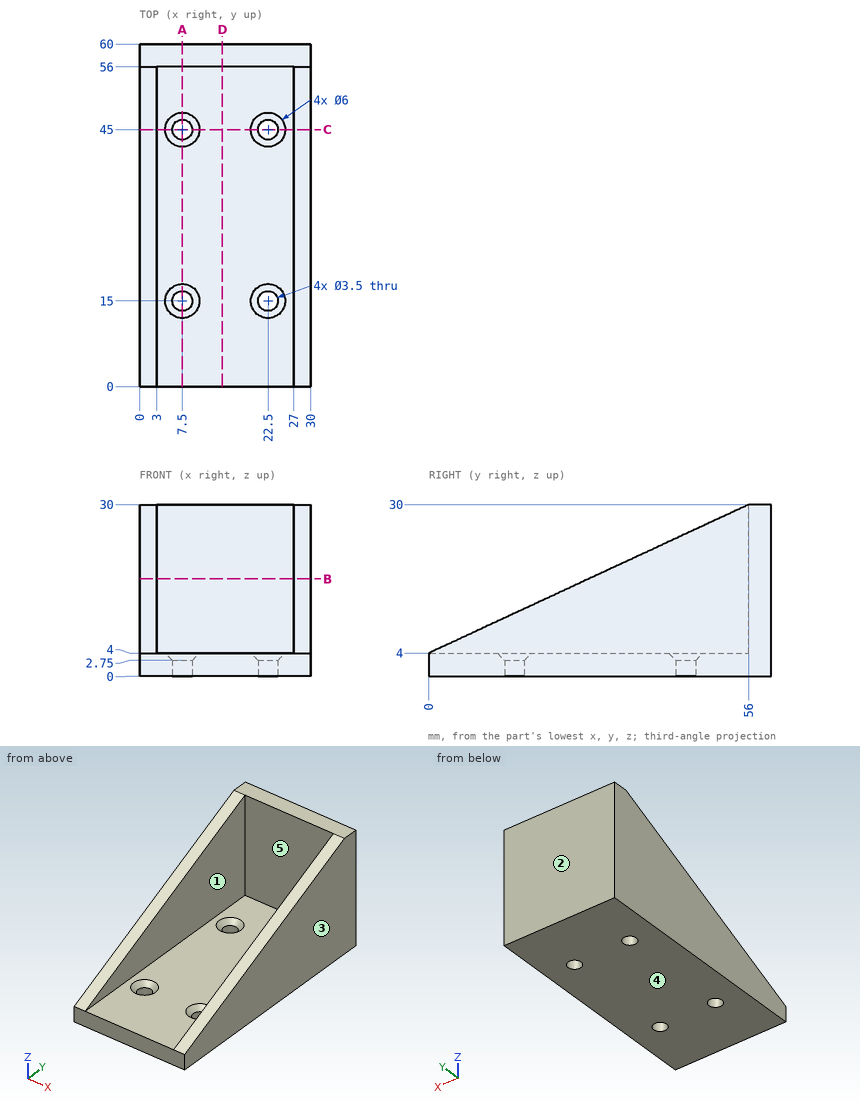
Here's the drawing with two shaded views (mm, measured from the low corner). I have some questions. A direction names the side the tool comes from. Coordinates: 2 decimals unless noted, no trailing zeros. Loops run counter-clockwise (first coordinate to the right, second up) from the corner with the lowest first, then second, coordinate; pieces in that order, holes last. Notation, with made-up numbers: (-3.75, 60.5) -> (14.25, 60.5) arc R35 cw to (14.25, 94.5) -> close; hole circle Ø8 at (83.25, 85). An arc over 180 degrees is marked (long way). Answer as a JSON object with one key per item and string values.
1) Imagine slicing it at D-D (x = 14.5). Please give me the cut outline in (y, z).
Results:
{"outline": "(0, 0) -> (60, 0) -> (60, 30) -> (56, 30) -> (56, 4) -> (0, 4) -> close"}
2) For the marked faces 4 and 5, which set-ups out of +Z, -Z, +X, -X, +Y, -Y let a thin tool reach every point of the face, with its end or its side?
Results:
{"face 4": "-Z, +X, -X, +Y, -Y", "face 5": "+Z, -Y"}
3) Imagine slicing it at C-C (y = 45). Please give me the cut outline in (x, z).
Results:
{"outline": "(0, 0) -> (5.75, 0) -> (5.75, 2.75) -> (4.5, 4) -> (3, 4) -> (3, 24.89) -> (0, 24.89) -> close; (9.25, 0) -> (20.75, 0) -> (20.75, 2.75) -> (19.5, 4) -> (10.5, 4) -> (9.25, 2.75) -> close; (24.25, 0) -> (30, 0) -> (30, 24.89) -> (27, 24.89) -> (27, 4) -> (25.5, 4) -> (24.25, 2.75) -> close"}
4) Imagine slicing it at B-B (z = 17). Please give me the cut outline in (x, y).
Results:
{"outline": "(0, 28) -> (3, 28) -> (3, 56) -> (27, 56) -> (27, 28) -> (30, 28) -> (30, 60) -> (0, 60) -> close"}
5) Thinking about a two-plate mould opening in X: for the marked faces 1, 2 and 3, which applies, pulls with the +X half, pulls with the -X half, needs draft (parallel to the pull), parting line crosses it, or undercut?
Results:
{"face 1": "undercut", "face 2": "needs draft", "face 3": "pulls with the +X half"}
6) Imagine slicing it at A-A (x = 7.5). Please give me the cut outline in (y, z), then the cut area to 3 significant figures.
Results:
{"outline": "(0, 0) -> (13.25, 0) -> (13.25, 2.75) -> (12, 4) -> (0, 4) -> close; (16.75, 0) -> (43.25, 0) -> (43.25, 2.75) -> (42, 4) -> (18, 4) -> (16.75, 2.75) -> close; (46.75, 0) -> (60, 0) -> (60, 30) -> (56, 30) -> (56, 4) -> (48, 4) -> (46.75, 2.75) -> close", "area": "313 mm^2"}
7) If I drill on line 1 (X direction, y = 15, z = 1.45); line 2 (Y direction, x = 7.5, z = 1.1); line 3 (X direction, y = 28, z = 14), over which ranges is the centre line in solid material (lowest first)?
Results:
{"line 1": "x = 0 to 5.75, 9.25 to 20.75, 24.25 to 30", "line 2": "y = 0 to 13.25, 16.75 to 43.25, 46.75 to 60", "line 3": "x = 0 to 3, 27 to 30"}
8) For P1, Ø8, axis at x = 17.5, z = 16.5, coming from the -Y side; P2, Ø1.5, axis at x = 26, y = 47.5, coming from the +Z side; P3, Ø3, axis at x = 22.5, y = 15, coming from the +Z side (1 decimal); P4, Ø4, axis at x = 7.5, y = 15, coming from the +Z side, each with a flat end and sliding along its axis, tell me the tip position at first contact or that it passes through.
Results:
{"P1": "stops at y = 56", "P2": "stops at z = 4", "P3": "passes through", "P4": "stops at z = 3"}
